from build123d import *

# Parameters (mm, degrees)
SKETCH2_R           = 110
SKETCH2_R_2         = 2
SKETCH2_R_3         = 3
BOSS_EXTRUDE1_DEPTH = 9
SKETCH4_R           = 2.5
CUT_EXTRUDE1_DEPTH  = 156.823618235


with BuildPart() as part:
    # Sketch2 → Boss-Extrude1 (new body)
    with BuildSketch(Plane(origin=(0, 0, 0), x_dir=(1, 0, 0), z_dir=(0, 1, 0))):
        with Locations(Location((0, 0, 0), (0, 0, 270))):
            Circle(SKETCH2_R)
        with Locations(Location((0, 74, 0), (0, 0, 270))):
            Circle(SKETCH2_R_2, mode=Mode.SUBTRACT)
        with Locations(Location((70.378182206, 22.867257584, 0), (0, 0, 270))):
            Circle(SKETCH2_R_2, mode=Mode.SUBTRACT)
        with Locations(Location((43.49610867, -59.867257584, 0), (0, 0, 270))):
            Circle(SKETCH2_R_2, mode=Mode.SUBTRACT)
        with Locations(Location((-43.49610867, -59.867257584, 0), (0, 0, 270))):
            Circle(SKETCH2_R_2, mode=Mode.SUBTRACT)
        with Locations(Location((-70.378182206, 22.867257584, 0), (0, 0, 270))):
            Circle(SKETCH2_R_2, mode=Mode.SUBTRACT)
        with Locations(Location((0, -72, 0), (0, 0, 270))):
            Circle(SKETCH2_R_3, mode=Mode.SUBTRACT)
        with Locations(Location((-68.476069173, -22.249223595, 0), (0, 0, 270))):
            Circle(SKETCH2_R_3, mode=Mode.SUBTRACT)
        with Locations(Location((-42.320538165, 58.249223595, 0), (0, 0, 270))):
            Circle(SKETCH2_R_3, mode=Mode.SUBTRACT)
        with Locations(Location((42.320538165, 58.249223595, 0), (0, 0, 270))):
            Circle(SKETCH2_R_3, mode=Mode.SUBTRACT)
        with Locations(Location((68.476069173, -22.249223595, 0), (0, 0, 270))):
            Circle(SKETCH2_R_3, mode=Mode.SUBTRACT)
        with BuildLine():
            ThreePointArc((-18.105238982, 77.924324324), (-23.772563309, 76.386289567), (-29.311797662, 74.436674548))
            ThreePointArc((-29.311797662, 74.436674548), (-32.653398245, 70.774561882), (-31.803317238, 65.890431875))
            ThreePointArc((-31.803317238, 65.890431875), (-34.679329885, 47.732002668), (-52.837759092, 50.608015315))
            ThreePointArc((-52.837759092, 50.608015315), (-57.220153284, 52.925769571), (-61.735640767, 50.879373611))
            ThreePointArc((-61.735640767, 50.879373611), (-65.301552386, 46.213712857), (-68.515609894, 41.299046004))
            ThreePointArc((-68.515609894, 41.299046004), (-68.964800278, 37.101160663), (-66.040677784, 34.055915028))
            ThreePointArc((-66.040677784, 34.055915028), (-58.96550401, 19.159053651), (-73.445595254, 11.265922437))
            ThreePointArc((-73.445595254, 11.265922437), (-77.601210519, 10.521023043), (-79.705262959, 6.860834978))
            ThreePointArc((-79.705262959, 6.860834978), (-79.99380451, 0.99561037), (-79.851327994, -4.87497873))
            ThreePointArc((-79.851327994, -4.87497873), (-77.401063247, -9.184684789), (-72.4932901, -9.885488883))
            ThreePointArc((-72.4932901, -9.885488883), (-56.112334461, -18.232002668), (-64.458848246, -34.612958307))
            ThreePointArc((-64.458848246, -34.612958307), (-68.017397816, -38.064637406), (-67.466521973, -42.991492331))
            ThreePointArc((-67.466521973, -42.991492331), (-64.131142201, -47.824644275), (-60.450214656, -52.400110191))
            ThreePointArc((-60.450214656, -52.400110191), (-56.59659591, -54.124533543), (-52.796791661, -52.284560445))
            ThreePointArc((-52.796791661, -52.284560445), (-36.442685642, -50.159053651), (-33.410466041, -66.369550469))
            ThreePointArc((-33.410466041, -66.369550469), (-33.986180358, -70.551962018), (-31.155322609, -73.684095116))
            ThreePointArc((-31.155322609, -73.684095116), (-25.666326768, -75.770968519), (-20.039037085, -77.449577098))
            ThreePointArc((-20.039037085, -77.449577098), (-15.183089607, -76.451009257), (-13, -72))
            ThreePointArc((-13, -72), (0, -59), (13, -72))
            ThreePointArc((13, -72), (15.183089607, -76.451009257), (20.039037085, -77.449577098))
            ThreePointArc((20.039037085, -77.449577098), (25.666326768, -75.770968519), (31.155322609, -73.684095116))
            ThreePointArc((31.155322609, -73.684095116), (33.986180358, -70.551962018), (33.410466041, -66.369550469))
            ThreePointArc((33.410466041, -66.369550469), (36.442685642, -50.159053651), (52.796791661, -52.284560445))
            ThreePointArc((52.796791661, -52.284560445), (56.59659591, -54.124533543), (60.450214656, -52.400110191))
            ThreePointArc((60.450214656, -52.400110191), (64.131142201, -47.824644275), (67.466521973, -42.991492331))
            ThreePointArc((67.466521973, -42.991492331), (68.017397816, -38.064637406), (64.458848246, -34.612958307))
            ThreePointArc((64.458848246, -34.612958307), (56.112334461, -18.232002668), (72.4932901, -9.885488883))
            ThreePointArc((72.4932901, -9.885488883), (77.401063247, -9.184684789), (79.851327994, -4.87497873))
            ThreePointArc((79.851327994, -4.87497873), (79.99380451, 0.99561037), (79.705262959, 6.860834978))
            ThreePointArc((79.705262959, 6.860834978), (77.601210519, 10.521023043), (73.445595254, 11.265922437))
            ThreePointArc((73.445595254, 11.265922437), (58.96550401, 19.159053651), (66.040677784, 34.055915028))
            ThreePointArc((66.040677784, 34.055915028), (68.964800278, 37.101160663), (68.515609894, 41.299046004))
            ThreePointArc((68.515609894, 41.299046004), (65.301552386, 46.213712857), (61.735640767, 50.879373611))
            ThreePointArc((61.735640767, 50.879373611), (57.220153284, 52.925769571), (52.837759092, 50.608015315))
            ThreePointArc((52.837759092, 50.608015315), (34.679329885, 47.732002668), (31.803317238, 65.890431875))
            ThreePointArc((31.803317238, 65.890431875), (32.653398245, 70.774561882), (29.311797662, 74.436674548))
            ThreePointArc((29.311797662, 74.436674548), (23.772563309, 76.386289567), (18.105238982, 77.924324324))
            ThreePointArc((18.105238982, 77.924324324), (13.974005311, 77.054311855), (11.98140815, 73.33227345))
            ThreePointArc((11.98140815, 73.33227345), (0, 62), (-11.98140815, 73.33227345))
            ThreePointArc((-11.98140815, 73.33227345), (-13.974005311, 77.054311855), (-18.105238982, 77.924324324))
        make_face(mode=Mode.SUBTRACT)
    extrude(amount=BOSS_EXTRUDE1_DEPTH)

    # Sketch4 → Cut-Extrude1 (cut, through all)
    with BuildSketch(Plane(origin=(0, 9, 0), x_dir=(1, 0, 0), z_dir=(0, 1, 0))):
        with Locations(Location((0, 74, 0), (0, 0, 270))):
            Circle(SKETCH4_R)
        with Locations(Location((70.378182206, 22.867257584, 0), (0, 0, 270))):
            Circle(SKETCH4_R)
        with Locations(Location((43.49610867, -59.867257584, 0), (0, 0, 270))):
            Circle(SKETCH4_R)
        with Locations(Location((-43.49610867, -59.867257584, 0), (0, 0, 270))):
            Circle(SKETCH4_R)
        with Locations(Location((-70.378182206, 22.867257584, 0), (0, 0, 270))):
            Circle(SKETCH4_R)
    extrude(amount=-CUT_EXTRUDE1_DEPTH, mode=Mode.SUBTRACT)


solid = part.part
Design review of the part built by this model. Coordinates are the model's own, in mm. Give positions to 0.01 mm unless a question says otherwise; leave off trailing zeros. Order: outer loops, then holes, each group sorted by start corner. A loop starts at its lowest first (then second) coordinate and runs counter-clockwise, first axis right, second up. Notation, with made-up numbers: (2, 86) - (59, 86) arc R15 ccw to (59, 91) - close; hole circle Ø1 at (4, 50). An arc over 180 degrees is marked (long way). Use CSV: the item, a comma, the result in double quotes. Start each with the question number.
Q1. Take a section at C-C (y = 3). Count the separate pieces of the cut face and the enclosed holes in it, and give its area (3 significant figures).
Q2. Take a section at A-A (z = 0). State the section outline as (x, y) points, and give its area (3 significant figures).
Q3. Draft analysis for pull direction Z (two halves, no side actions). For faces 1 (the face through (42.539, 4.563, 62.177)), 2 (the face through (-47, 0, -50)), 3 (the face through (56.536, 4.437, 54.123)), state which applies: pulls with the +Z half, pulls with the -Z half, needs draft (parallel to the pull), parting line crosses it, or undercut.
Q4. For line 1 (X direction, y = 5, z = -74); line 2 (Z direction, x = 57, y = 5); line 3 (X direction, y = 4.5, z = -1), list the stretches that pass through material, from the lowest coordinate up.
Q5. For P1, Ø5, axis at y = 1.5, z = -50.5, coming from the +X side; P2, Ø1, axis at y = 5, z = -56.5, coming from the +X side; P3, Ø5, axis at x = 42.32, z = -58.25, coming from the -Y side; P4, Ø2, axis at y = 2.5, z = -46.5, coming from the -X side, all flat-tipped, find the tip position at first contact; note any pin that passes through.
Q6. Take a section at B-B (x = 0). State the section outline as (y, z) points.
Calculated:
1,separate pieces,"1"
1,enclosed holes,"11"
1,area,"22,000 mm²"
2,outline,"(-110, 0) - (-80, 0) - (-80, 9) - (-110, 9) - close; (80, 0) - (110, 0) - (110, 9) - (80, 9) - close"
2,area,"540 mm²"
3,face 1,"undercut"
3,face 2,"needs draft"
3,face 3,"undercut"
4,line 1,"x = -81.39 to -30.19, -12.06 to -2.5, 2.5 to 12.06, 30.19 to 81.39"
4,line 2,"z = -94.08 to -52.91, 16.14 to 28.36, 54.11 to 94.08"
4,line 3,"x = -110 to -79.99, 79.99 to 110"
5,P1,"stops at x = 98.97"
5,P2,"stops at x = 94.68"
5,P3,"passes through"
5,P4,"stops at x = -100.15"
6,outline,"(0, -110) - (9, -110) - (9, -76.5) - (0, -76.5) - close; (0, -71.5) - (9, -71.5) - (9, -62) - (0, -62) - close; (0, 59) - (9, 59) - (9, 69) - (0, 69) - close; (0, 75) - (9, 75) - (9, 110) - (0, 110) - close"
